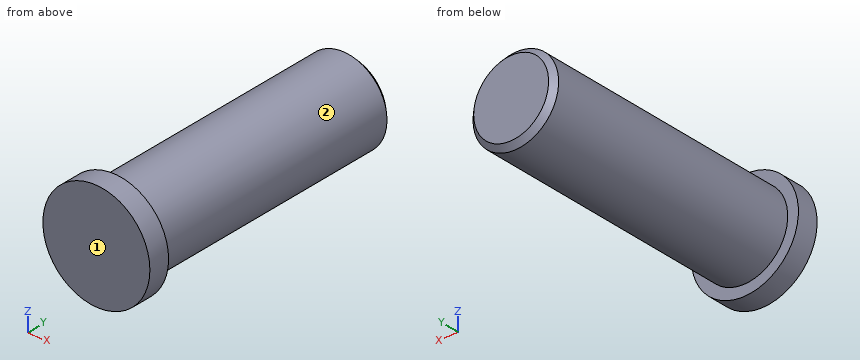
from build123d import *

# Parameters (mm, degrees)
SKETCH1_R           = 5
BOSS_EXTRUDE1_DEPTH = 2
SKETCH2_R           = 4
BOSS_EXTRUDE2_DEPTH = 25
CHAMFER1_SIZE       = 0.5


with BuildPart() as part:
    # Sketch1 → Boss-Extrude1 (new body)
    with BuildSketch(Plane(origin=(0, 0, 0), x_dir=(1, 0, 0), z_dir=(0, 1, 0))):
        Circle(SKETCH1_R)
    extrude(amount=BOSS_EXTRUDE1_DEPTH)

    # Sketch2 → Boss-Extrude2 (add)
    with BuildSketch(Plane(origin=(0, 2, 0), x_dir=(1, 0, 0), z_dir=(0, 1, 0))):
        Circle(SKETCH2_R)
    extrude(amount=BOSS_EXTRUDE2_DEPTH)

    # Chamfer1
    chamfer1_edges = [part.edges().sort_by_distance(p)[0] for p in [
        (-4, 27, 0),
    ]]
    chamfer(chamfer1_edges, length=CHAMFER1_SIZE)


solid = part.part
Geometry check sheet. Reference: the model listing, model coordinates, mm. Face numbers are marked on the shaded views. A direction names the side the tool comes from. Give positions to 0.01 mm unless a question says otherwise; leave off trailing zeros. Order: outer loops, then holes, each group sorted by start corner. A loop starts at its lowest first (then second) coordinate and runs counter-clockwise, first axis right, second up. Notation, with made-up numbers: (33, -24.75) - (51, -24.75) arc R22 cw to (51, 12.25) - close; hole circle Ø5 at (73, 85.5). An arc over 180 degrees is marked (long way). Use one line per item in the form item = value.
1) Sectioned sample at B-B (x = 0). Record the boundary of the cut face in (y, z), and give its area (3 significant figures).
Working result:
outline = (0, -5) - (2, -5) - (2, -4) - (26.5, -4) - (27, -3.5) - (27, 3.5) - (26.5, 4) - (2, 4) - (2, 5) - (0, 5) - close
area = 220 mm^2
2) Access from +Z, -Z, +X, -X, +Y, -Y to the whole of each face (thin tool, end or side, straight path). Record for the marked faces 1 and 2.
Working result:
face_1 = +Z, -Z, +X, -X, -Y
face_2 = +Y
3) Sectioned sample at A-A (z = 0). Record the boundary of the cut face in (x, y), and give its area (3 significant figures).
Working result:
outline = (-5, 0) - (5, 0) - (5, 2) - (4, 2) - (4, 26.5) - (3.5, 27) - (-3.5, 27) - (-4, 26.5) - (-4, 2) - (-5, 2) - close
area = 220 mm^2
4) Material ranges on probe 1 along Y at (x, z) = (-1, 4.5); probe 2 along Z at (x, y) = (3, 13.75); probe 3 along Z at (x, y) = (-2.5, 3), recorded low to high. Write a range as from..to.
Working result:
probe_1 = 0..2
probe_2 = -2.65..2.65
probe_3 = -3.12..3.12
5) Depth check by flat-ended pin: pin 1 Ø6 at (x, y) = (-4, 12.5) entering from +Z; pin 2 Ø2 at (y, z) = (10, -4) entering from -X. Enter the tip coordinate at first touch or a pass-through.
Working result:
pin_1 = 3.87
pin_2 = -2.65
6) Sectioned sample at C-C (y = 19). Record the boundary of the cut face in (x, z).
Working result:
outline = circle Ø8 at (0, 0)
